Build history of the part. All positions in model axes, mm. A direction names the side the tool comes from. Give positions to 0.01 mm unless a question says otherwise; leave off trailing zeros. Order: outer loops, then holes, each group sorted by start corner. A loop starts at its lowest first (then second) coordinate and runs counter-clockwise, first axis right, second up. Notation, with made-up numbers: M 47.25,-12.5 L 51.25,-12.5 A23 ccw 51.25,1.5 Z; hole C -14,-13 d5. An arc over 180 degrees is marked long. Answer as CSV lines item,"result".
from build123d import *

# Parameters (mm, degrees)
SKETCH1_W           = 34.5
SKETCH1_H           = 49.5
BOSS_EXTRUDE1_DEPTH = 8
SKETCH2_R           = 3.1
CUT_EXTRUDE1_DEPTH  = 61.864603835
SKETCH3_W           = 6
SKETCH3_H           = 25
BOSS_EXTRUDE2_DEPTH = 8
FILLET1_R           = 10
FILLET2_R           = 5
BOSS_EXTRUDE3_DEPTH = 8
SKETCH8_R           = 2.25
CUT_EXTRUDE2_DEPTH  = 202.585744784


with BuildPart() as part:
    # Sketch1 → Boss-Extrude1 (new body)
    with BuildSketch(Plane(origin=(0, 0, 0), x_dir=(1, 0, 0), z_dir=(0, 1, 0))):
        with Locations((17.25, 24.75)):
            Rectangle(SKETCH1_W, SKETCH1_H)
    extrude(amount=BOSS_EXTRUDE1_DEPTH)

    # Sketch2 → Cut-Extrude1 (cut, through all)
    with BuildSketch(Plane(origin=(0, 8, 0), x_dir=(1, 0, 0), z_dir=(0, 1, 0))):
        with Locations(Location((5, 39.75, 0), (0, 0, 270))):
            Circle(SKETCH2_R)
        with Locations(Location((5, 9.75, 0), (0, 0, 90))):
            Circle(SKETCH2_R)
        with Locations(Location((29.5, 9.75, 0), (0, 0, 270))):
            Circle(SKETCH2_R)
        with Locations(Location((29.5, 39.75, 0), (0, 0, 90))):
            Circle(SKETCH2_R)
    extrude(amount=-CUT_EXTRUDE1_DEPTH, mode=Mode.SUBTRACT)

    # Sketch3 → Boss-Extrude2 (add, through all)
    with BuildSketch(Plane(origin=(0, 8, 0), x_dir=(1, 0, 0), z_dir=(0, 1, 0))):
        Polygon((195.25, 42.25), (34.5, 49.5), (34.5, 41.491867701), (89.599952536, 39.006799857), (89.599952536, 10.493200143), (34.5, 8.008132299), (34.5, 0), (195.25, 7.25), align=None)
        Polygon((176.564901879, 14.415414033), (94.599952536, 10.718705586), (94.599952536, 38.781294414), (176.564901879, 35.084585967), align=None, mode=Mode.SUBTRACT)
        with Locations((186.63, 24.75)):
            Rectangle(SKETCH3_W, SKETCH3_H, mode=Mode.SUBTRACT)
    extrude(amount=-BOSS_EXTRUDE2_DEPTH)

    # Fillet1
    fillet1_edges = [part.edges().sort_by_distance(p)[0] for p in [
        (34.5, 4, -8.008132299),
        (89.599952536, 4, -10.493200143),
        (89.599952536, 4, -39.006799857),
        (34.5, 4, -41.491867701),
        (94.599952536, 4, -38.781294414),
        (94.599952536, 4, -10.718705586),
    ]]
    fillet(fillet1_edges, radius=FILLET1_R)

    # Fillet2
    fillet2_edges = [part.edges().sort_by_distance(p)[0] for p in [
        (176.564901879, 4, -35.084585967),
        (176.564901879, 4, -14.415414033),
    ]]
    fillet(fillet2_edges, radius=FILLET2_R)

    # Sketch7 → Boss-Extrude3 (add, through all)
    with BuildSketch(Plane(origin=(0, 8, 0), x_dir=(1, 0, 0), z_dir=(0, 1, 0))):
        with BuildLine():
            Line((105.050505418, 11.190036898), (171.79017832, 14.200068802))
            ThreePointArc((171.79017832, 14.200068802), (175.179205561, 15.740022551), (176.564901879, 19.194991277))
            Line((176.564901879, 19.194991277), (176.564901879, 30.305008723))
            ThreePointArc((176.564901879, 30.305008723), (175.179205561, 33.759977449), (171.79017832, 35.299931198))
            Line((171.79017832, 35.299931198), (105.050505418, 38.309963102))
            ThreePointArc((105.050505418, 38.309963102), (97.690015084, 35.548725516), (94.599952536, 28.320118153))
            Line((94.599952536, 28.320118153), (94.599952536, 21.179881847))
            ThreePointArc((94.599952536, 21.179881847), (97.690015084, 13.951274484), (105.050505418, 11.190036898))
        make_face()
        with BuildLine():
            Line((89.599952536, 20.052354631), (89.599952536, 29.447645369))
            ThreePointArc((89.599952536, 29.447645369), (86.828559899, 36.357582821), (80.050505418, 39.437490318))
            Line((80.050505418, 39.437490318), (44.950552883, 41.020536389))
            ThreePointArc((44.950552883, 41.020536389), (37.590062548, 38.259298803), (34.5, 31.03069144))
            Line((34.5, 31.03069144), (34.5, 18.46930856))
            ThreePointArc((34.5, 18.46930856), (37.590062548, 11.240701197), (44.950552883, 8.479463611))
            Line((44.950552883, 8.479463611), (80.050505418, 10.062509682))
            ThreePointArc((80.050505418, 10.062509682), (86.828559899, 13.142417179), (89.599952536, 20.052354631))
        make_face()
    extrude(amount=-BOSS_EXTRUDE3_DEPTH)

    # Sketch8 → Cut-Extrude2 (cut, through all)
    with BuildSketch(Plane(origin=(0, 8, 0), x_dir=(1, 0, 0), z_dir=(0, 1, 0))):
        with Locations(Location((163.63, 33.5, 0), (0, 0, 270))):
            Circle(SKETCH8_R)
        with Locations(Location((163.63, 16, 0), (0, 0, 270))):
            Circle(SKETCH8_R)
    extrude(amount=-CUT_EXTRUDE2_DEPTH, mode=Mode.SUBTRACT)


solid = part.part
Item 1: Probe line 1 along Z through (x, y) = (30, 1); line 2 along X through (y, z) = (5, -16); line 3 along X through (y, z) = (1.75, -39.75). List the from-to ranges inside material, lowest first. Write a range as from..to.
Geometry says:
line 1,"z = -49.5..-42.81, -36.69..-12.81, -6.69..0"
line 2,"x = 0..161.38, 165.88..183.63, 189.63..195.25"
line 3,"x = 0..1.9, 8.1..26.4, 32.6..195.25"
Item 2: Band-saw the part on D-D (y = 4.25). Give the cut face in (x, z), and give its area (3 significant figures).
Geometry says:
outline,"M 0,-49.5 L 34.5,-49.5 L 195.25,-42.25 L 195.25,-7.25 L 34.5,0 L 0,0 Z; hole C 5,-39.75 d6.2; hole C 5,-9.75 d6.2; hole C 29.5,-39.75 d6.2; hole C 29.5,-9.75 d6.2; hole C 163.63,-33.5 d4.5; hole C 163.63,-16 d4.5; hole M 183.63,-37.25 L 189.63,-37.25 L 189.63,-12.25 L 183.63,-12.25 Z"
area,"8,200 mm2"
Item 3: Band-saw the part on B-B (x = 5). Give the cut face in (y, z), and give its area (3 significant figures).
Geometry says:
outline,"M 0,-49.5 L 8,-49.5 L 8,-42.85 L 0,-42.85 Z; M 0,-36.65 L 8,-36.65 L 8,-12.85 L 0,-12.85 Z; M 0,-6.65 L 8,-6.65 L 8,0 L 0,0 Z"
area,"297 mm2"
Item 4: Pull direction Z, two halves, no side cores. Call faces 3 (the flat face through (96, 0, -25)), 4 (the flat face through (17, 4, 0)), 5 (the flat face through (189.63, 4, -25)): released by +Z, released by -Z, zero draft, split by the parting line, or undercut.
Geometry says:
face 3,"zero draft"
face 4,"released by +Z"
face 5,"undercut"
Item 5: Band-saw the part on A-A (z = -9.75). Give the cut face in (x, y).
Geometry says:
outline,"M 0,0 L 1.9,0 L 1.9,8 L 0,8 Z; M 8.1,0 L 26.4,0 L 26.4,8 L 8.1,8 Z; M 32.6,0 L 195.25,0 L 195.25,8 L 32.6,8 Z"
Item 6: 3-axis set-ups, long thin cutter, end or side, ignore diameter. For faces 1 (the flat face through (0, 4, -24)), 2 (the flat face through (187, 4, -12.25)): which of +Z, -Z, +X, -X, +Y, -Y reach the whole face in a straight line?
Geometry says:
face 1,"+Z, -Z, -X, +Y, -Y"
face 2,"+Y, -Y"
Item 7: Drop a flat-ended pin along its axis: pin 1 (1.5 mm diameter, centred on x = 61, y = 2, fed in from -Z). Give the stop position or say it passes through.
Geometry says:
pin 1,"stops at z = -48.34"
Item 8: Band-saw the part on C-C (z = -29). Give the cut face in (x, y), and give its area (3 significant figures).
Geometry says:
outline,"M 0,0 L 183.63,0 L 183.63,8 L 0,8 Z; M 189.63,0 L 195.25,0 L 195.25,8 L 189.63,8 Z"
area,"1,510 mm2"
